```python
from build123d import *

# Parameters (mm, degrees)
CROQUIS1_R              = 48
CROQUIS1_R_2            = 13.5
SALIENTE_EXTRUIR3_DEPTH = 10
TALADRO1_D              = 11
TALADRO1_DEPTH          = 100
TALADRO1_CBORE_D        = 18
TALADRO1_CBORE_DEPTH    = 3
TALADRO1_TIP            = 3.304733405
CROQUIS9_R              = 18
CROQUIS9_R_2            = 13.5
CROQUIS15_R             = 48
CROQUIS15_R_2           = 13.5
SALIENTE_EXTRUIR5_DEPTH = 10
TALADRO3_AT_2_COUNT     = 2
TALADRO3_AT_2_PITCH     = 42.426406871
TALADRO3_AT_3_COUNT     = 2
TALADRO3_AT_3_PITCH     = 60
TALADRO3_AT_4_COUNT     = 2
TALADRO3_AT_4_PITCH     = 42.426406871


with BuildPart() as part:
    # Croquis1 → Saliente-Extruir3 (new body)
    with BuildSketch(Plane(origin=(0, 0, 0), x_dir=(1, 0, 0), z_dir=(0, 1, 0))):
        Circle(CROQUIS1_R)
        Circle(CROQUIS1_R_2, mode=Mode.SUBTRACT)
    extrude(amount=SALIENTE_EXTRUIR3_DEPTH)

    # Taladro1
    with Locations(Plane(origin=(0, 10, 0), x_dir=(1, 0, 0), z_dir=(0, 1, 0))):
        with Locations((-33, 0), (0, 33), (33, 0), (0, -33)):
            CounterBoreHole(TALADRO1_D / 2, TALADRO1_CBORE_D / 2, TALADRO1_CBORE_DEPTH, depth=TALADRO1_DEPTH)
            with Locations((0, 0, -(TALADRO1_DEPTH + TALADRO1_TIP / 2))):  # 118° drill point
                Cone(0, TALADRO1_D / 2, TALADRO1_TIP, mode=Mode.SUBTRACT)

    # Barrer2: sweep along a path in Croquis14
    with BuildLine(Plane(origin=(0, 0, 0), x_dir=(0, 0, -1), z_dir=(1, 0, 0))) as barrer2_path:
        ThreePointArc((0, 10), (-39.065769178, 149.354207944), (-182.805987365, 166.220721172))
    # Croquis9 → Barrer2 (sweep)
    with BuildSketch(Plane(origin=(0, 10, 0), x_dir=(1, 0, 0), z_dir=(0, 1, 0))):
        Circle(CROQUIS9_R)
        Circle(CROQUIS9_R_2, mode=Mode.SUBTRACT)
    sweep(path=barrer2_path.line)

    # Croquis15 → Saliente-Extruir5 (add)
    with BuildSketch(Plane(origin=(0, -7.432010892, 7.35587441), x_dir=(1, 0, 0), z_dir=(0, -0.710737951, 0.703456868))):
        with Locations((0, 246.856260786)):
            Circle(CROQUIS15_R)
        with Locations((0, 246.856260786)):
            Circle(CROQUIS15_R_2, mode=Mode.SUBTRACT)
    extrude(amount=SALIENTE_EXTRUIR5_DEPTH)

    # Croquis21 → Taladro3 (revolve, cut)
    with BuildSketch(Plane(origin=(30, 168.331091776, 184.938201218), x_dir=(0, 0.703456868, 0.710737951), z_dir=(1, 0, 0))):
        Polygon((0, 0), (0, 103.304733405), (5.5, 100), (5.5, 3), (9, 3), (9, 0), align=None)
    taladro3 = revolve(axis=Axis((30, 176.370159924, 176.981488488), (0, -0.710737951, 0.703456868)), mode=Mode.SUBTRACT)

    # Taladro3 at 2: Taladro3 ×2
    with Locations(*[Vector(-0.707106781, 0.497419122, 0.502567625) * (i * TALADRO3_AT_2_PITCH) for i in range(1, TALADRO3_AT_2_COUNT)]):
        add(taladro3, mode=Mode.SUBTRACT)

    # Taladro3 at 3: Taladro3 ×2
    with Locations(*[(-i * TALADRO3_AT_3_PITCH, 0, 0) for i in range(1, TALADRO3_AT_3_COUNT)]):
        add(taladro3, mode=Mode.SUBTRACT)

    # Taladro3 at 4: Taladro3 ×2
    with Locations(*[Vector(-0.707106781, -0.497419122, -0.502567625) * (i * TALADRO3_AT_4_PITCH) for i in range(1, TALADRO3_AT_4_COUNT)]):
        add(taladro3, mode=Mode.SUBTRACT)


solid = part.part
```
Can you work these out from the model? Positions are in its coordinate system, mm. A direction names the side the tool comes from. Round coordinates to 2 decimals unless told otherwise and drop trailing zeros. Loops run counter-clockwise (first coordinate to the right, second up) from the corner with the lowest first, then second, coordinate; pieces in that order, holes last. Notation, with made-up numbers: (34.5, -19) -> (49.5, -19) arc R31 ccw to (49.5, 10) -> close; hole circle Ø8 at (67.25, -25). An arc over 180 degrees is marked (long way). Answer in a Markdown table with one row per item.
Item 1: On a 3-axis mill with a long thin cutter (end or side, diameter ignored), from which of +Z, -Z, +X, -X, +Y, -Y can I reach the whole of each face in a straight line? I mean faces 1 (the cylindrical face through (0.716, 3.451, 27.547)), 2 (the flat face through (3.9, 190.2, 211.3)), 3 (the flat face through (10, 0, 10)), 4 (the cylindrical face through (-42, 9, 0)), 5 (the cylindrical face through (0.716, 3.451, -38.453)). Say none if no direction works.
Answer block:
| item | result |
|---|---|
| face 1 | -Y |
| face 2 | none |
| face 3 | +Z, -Z, +X, -X, -Y |
| face 4 | +Y |
| face 5 | +Y, -Y |
Item 2: If I drill on probe 1 along Z at (x, y) = (0, 8); probe 2 along Z at (x, y) = (0, 4.5); probe 3 along Z at (x, y) = (4, 134), over which ranges is the centre line in solid material (lowest first)?
Answer block:
| item | result |
|---|---|
| probe 1 | -48 to -42, -24 to -13.5, 13.5 to 24, 42 to 48 |
| probe 2 | -48 to -38.5, -27.5 to -13.5, 13.5 to 27.5, 38.5 to 48 |
| probe 3 | 2.79 to 8.27, 40.38 to 46.68, 150.25 to 164.47 |
Item 3: Suppose I cut it at A-A, the plane z = -33. List the corners of the cut face in (x, y) for me.
Answer block:
| item | result |
|---|---|
| outline | (-34.86, 0) -> (-5.5, 0) -> (-5.5, 7) -> (-9, 7) -> (-9, 10) -> (-34.86, 10) -> close; (5.5, 0) -> (34.86, 0) -> (34.86, 10) -> (9, 10) -> (9, 7) -> (5.5, 7) -> close |
Item 4: Suppose I cut it at B-B, the plane z = 0. Give the number of separate pieces and of enclosed holes in the cut face, plus the area to 3 significant figures.
Answer block:
| item | result |
|---|---|
| separate pieces | 3 |
| enclosed holes | 0 |
| area | 1,670 mm² |
Item 5: Will these pins go through, and if not, where does the flat tip stop? P1, Ø3, axis at x = -3.5, z = 170.5, coming from the +Y side; P2, Ø21.5, axis at x = 0, z = 0, coming from the +Y side; P3, Ø14.5, axis at x = 0, z = 33, coming from the +Y side.
Answer block:
| item | result |
|---|---|
| P1 | y = 190.26 |
| P2 | y = 145.15 |
| P3 | y = 171.92 |
Item 6: We'd pull the mould along Z, two halves only. Please class faces 6 (the flat face through (9.995, 152.083, 182.737)), 7 (the cylindrical face through (-47.954, 4.93, -2.11)), 8 (the cylindrical face through (-2.93, 4.93, 13.18)), 9 (the flat face through (21, 10, -1)): released by +Z, released by -Z, zero draft, split by the parting line, or undercut.
Answer block:
| item | result |
|---|---|
| face 6 | released by +Z |
| face 7 | split by the parting line |
| face 8 | undercut |
| face 9 | zero draft |
